Here's how the part is built. I have some questions about the finished solid (model axes, mm). A direction names the side the tool comes from. Coordinates: 2 decimals unless noted, no trailing zeros. Write each loop counter-clockwise with the first axis right and the second up, starting at its lowest first coordinate (ties: lowest second). Pieces come first, ordered by that corner, then holes. Notation, with made-up numbers: (34, -12.75) -> (59, -12.75) arc R26 cw to (59, 21.25) -> close; hole circle Ø9 at (51, 19.25). An arc over 180 degrees is marked (long way). Use a Markdown table: item, result. Add a question column.
Item 1: If we mould it in two halves opening along Y, with no side actions, what happens to faces 1 (the flat face through (0, 30, 7)), 2 (the flat face through (-8, 19, 11)), 3 (the cylindrical face through (6.301, 22.146, 9.84)), 4 (the cylindrical face through (0.62, 24.72, 7.4))? For each: pulls with the +Y half, pulls with the -Y half, needs draft (parallel to the pull), parting line crosses it, or undercut.
Item 2: Imagine slicing it at B-B, the plane x = 0. Write out the boundary of the cut face in (y, z).
Item 3: If I drill on line 1 along Y through (x, z) = (-6.25, 7.5) (3 decimals); line 2 along Z through (x, y) = (5.1, 20) (3 decimals); line 3 along Y through (x, z) = (-2, 11.5), over which ranges is the centre line in solid material (lowest first)? Write a range as from..to.
Item 4: Will these pins go through, and if not, where does the flat tip stop? pin 1 Ø3 at (x, z) = (4.5, 13) entering from -Y; pin 2 Ø6 at (x, y) = (-1.5, -1) entering from +Z; pin 3 Ø7 at (x, z) = (2.5, 4) entering from -Y.
Item 5: On a 3-axis mill with a long thin cutter (end or side, diameter ignored), from which of +Z, -Z, +X, -X, +Y, -Y can I reach the whole of each face in a straight line? I mean faces 5 (the cylindrical face through (-6.238, 22.677, 5.793)), 6 (the flat face through (0, 12, 4)). Say none if no direction works.
Item 6: Imagine slicing it at D-D, the plane z = 2.25. Write out the boundary of the cut face in (x, y) (1 decimal).
Item 7: Imagine slicing it at C-C, the plane y = 20. Write out the boundary of the cut face in (x, z) (1 decimal).
Item 8: Imagine slicing it at A-A, the plane z = 7.5. Write out the boundary of the cut face in (x, y) (1 decimal), and give its area (3 significant figures).
```python
from build123d import *

# Parameters (mm, degrees)
SKETCH1_R                  = 2.5
BOSS_EXTRUDE1_DEPTH        = 15
SKETCH6_W                  = 16
SKETCH6_H                  = 20
CUT_EXTRUDE1_DEPTH         = 9
FILLET1_R                  = 2.5
F_3_8_0_3750_DOWEL_HOLE1_D = 9.525
F_1_4_0_2500_DOWEL_HOLE2_D = 6.35


with BuildPart() as part:
    # Sketch1 → Boss-Extrude1 (new body)
    with BuildSketch(Plane.XY):
        with BuildLine():
            Line((-8, 12), (-8, 0))
            ThreePointArc((-8, 0), (0, -8), (8, 0))
            Line((8, 0), (8, 12))
            Line((8, 12), (8, 30))
            Line((8, 30), (-8, 30))
            Line((-8, 30), (-8, 12))
        make_face()
        Circle(SKETCH1_R, mode=Mode.SUBTRACT)
    extrude(amount=BOSS_EXTRUDE1_DEPTH)

    # Sketch6 → Cut-Extrude1 (cut)
    with BuildSketch(Plane.XY):
        with Locations((0, 2)):
            Rectangle(SKETCH6_W, SKETCH6_H)
    extrude(amount=CUT_EXTRUDE1_DEPTH, mode=Mode.SUBTRACT)

    # Fillet1
    fillet1_edges = [part.edges().sort_by_distance(p)[0] for p in [
        (-2.5, 0, 15),
        (-2.5, 0, 9),
    ]]
    fillet(fillet1_edges, radius=FILLET1_R)

    # 3/8 (0.3750) Dowel Hole1 (through all)
    with Locations(Plane.XY.offset(15)):
        with Locations((0, 20)):
            Hole(F_3_8_0_3750_DOWEL_HOLE1_D / 2)

    # 1/4 (0.2500) Dowel Hole2 (through all)
    with Locations(Plane.ZY.offset(8)):
        with Locations((7.5, 20)):
            Hole(F_1_4_0_2500_DOWEL_HOLE2_D / 2)


solid = part.part
```
Ans:
| question | item | result |
|---|---|---|
| 1 | face 1 | pulls with the +Y half |
| 1 | face 2 | needs draft |
| 1 | face 3 | undercut |
| 1 | face 4 | undercut |
| 2 | outline | (-8, 9) -> (-5, 9) arc R2.5 ccw to (-2.5, 11.5) -> (-2.5, 12.5) arc R2.5 ccw to (-5, 15) -> (-8, 15) -> close; (2.5, 11.5) arc R2.5 ccw to (5, 9) -> (12, 9) -> (12, 0) -> (15.24, 0) -> (15.24, 15) -> (5, 15) arc R2.5 ccw to (2.5, 12.5) -> close; (24.76, 0) -> (30, 0) -> (30, 15) -> (24.76, 15) -> close |
| 3 | line 1 | y = 12..16.825, 23.175..30 |
| 3 | line 2 | z = 0..4.325, 10.675..15 |
| 3 | line 3 | y = -7.75..-1.5, 1.5..15.68, 24.32..30 |
| 4 | pin 1 | stops at y = -7.42 |
| 4 | pin 2 | stops at z = 14.99 |
| 4 | pin 3 | stops at y = 12 |
| 5 | face 5 | +X, -X |
| 5 | face 6 | -Z, +X, -X, -Y |
| 6 | outline | (-8, 12) -> (8, 12) -> (8, 30) -> (-8, 30) -> close; hole circle Ø9.5 at (0, 20) |
| 7 | outline | (-8, 0) -> (-4.8, 0) -> (-4.8, 4.3) -> (-8, 4.3) -> close; (-8, 10.7) -> (-4.8, 10.7) -> (-4.8, 15) -> (-8, 15) -> close; (4.8, 0) -> (8, 0) -> (8, 4.3) -> (4.8, 4.3) -> close; (4.8, 10.7) -> (8, 10.7) -> (8, 15) -> (4.8, 15) -> close |
| 8 | outline | (-8, 12) -> (8, 12) -> (8, 16.8) -> (3.5, 16.8) arc R4.8 cw to (-3.5, 16.8) -> (-8, 16.8) -> close; (-8, 23.2) -> (-3.5, 23.2) arc R4.8 cw to (3.5, 23.2) -> (8, 23.2) -> (8, 30) -> (-8, 30) -> close |
| 8 | area | 171 mm^2 |
